```python
from build123d import *

# Parameters (mm, degrees)
SKETCH1_R               = 6.35
BOSS_EXTRUDE1_DEPTH     = 17.5
CUT_EXTRUDE1_DEPTH      = 13
CHAMFER1_SIZE           = 2
SKETCH4_R               = 3.5
BOSS_EXTRUDE2_DEPTH     = 25
SKETCH6_R               = 1.75
CUT_EXTRUDE2_DEPTH      = 30
SKETCH7_R               = 2.5
CUT_EXTRUDE3_DEPTH      = 3.5
CUT_EXTRUDE4_DEPTH      = 101.436547133
CUT_EXTRUDE4_DEPTH_BACK = 101.436547133
SKETCH8_W               = 138.060190548
SKETCH8_H               = 48.357154547
SKETCH9_R               = 6.935
CUT_EXTRUDE5_DEPTH      = 1
MIRROR1_START           = -12.5
MIRROR1_OUTLINE_R       = 1.75
MIRROR1_DEPTH           = 25
MIRROR1_START_2         = -17.5
MIRROR1_2_OUTLINE_R     = 2.5
MIRROR1_2_DEPTH         = 3.5
MIRROR1_START_3         = -14
MIRROR1_3_OUTLINE_R     = 1.75
MIRROR1_3_DEPTH         = 1.5
MIRROR1_4_OUTLINE_R     = 6.935
MIRROR1_4_OUTLINE_R_2   = 6.35
MIRROR1_4_DEPTH         = 1
CUT_EXTRUDE6_DEPTH      = 101.436547133
CUT_EXTRUDE6_DEPTH_BACK = 101.436547133
SKETCH10_W              = 1
SKETCH10_H              = 7.5


# Read off the part's stored shape, not the designer's step: Mirror1
with BuildPart() as part:
    # Sketch1 → Boss-Extrude1 (new, symmetric)
    with BuildSketch(Plane(origin=(0, 0, 0), x_dir=(0, 0, -1), z_dir=(1, 0, 0))):
        with BuildLine():
            Line((-75, -17.5), (75, -17.5))
            ThreePointArc((75, -17.5), (91.201851746, -6.614378278), (87.247448714, 12.5))
            Line((87.247448714, 12.5), (-87.247448714, 12.5))
            ThreePointArc((-87.247448714, 12.5), (-91.201851746, -6.614378278), (-75, -17.5))
        make_face()
        with Locations((-75, 0)):
            Circle(SKETCH1_R, mode=Mode.SUBTRACT)
        with Locations((75, 0)):
            Circle(SKETCH1_R, mode=Mode.SUBTRACT)
    extrude(amount=BOSS_EXTRUDE1_DEPTH, both=True)

    # Sketch3 → Cut-Extrude1 (cut, symmetric)
    with BuildSketch(Plane(origin=(0, 0, 0), x_dir=(0, 0, -1), z_dir=(1, 0, 0))):
        with BuildLine():
            Line((-92.5, 12.5), (75, 12.5))
            ThreePointArc((75, 12.5), (87.5, 0), (75, -12.5))
            Line((75, -12.5), (-55, -12.5))
            Line((-55, -12.5), (-55, -17.5))
            Line((-55, -17.5), (-92.5, -17.5))
            Line((-92.5, -17.5), (-92.5, 12.5))
        make_face()
    extrude(amount=CUT_EXTRUDE1_DEPTH, both=True, mode=Mode.SUBTRACT)

    # Chamfer1
    chamfer1_edges = [part.edges().sort_by_distance(p)[0] for p in [
        (17.5, -6.614378278, -91.201851746),
        (0, -12.5, 55),
        (17.5, -6.614378278, 91.201851746),
        (-17.5, -6.614378278, -91.201851746),
        (-17.5, -17.5, 0),
        (-17.5, -6.614378278, 91.201851746),
        (17.5, -17.5, 0),
    ]]
    chamfer(chamfer1_edges, length=CHAMFER1_SIZE)

    # Sketch4 → Boss-Extrude2 (add)
    with BuildSketch(Plane(origin=(0, -12.5, 0), x_dir=(1, 0, 0), z_dir=(0, 1, 0))):
        with Locations((-10, 62.5)):
            Circle(SKETCH4_R)
        with Locations((-10, 26.333333333)):
            Circle(SKETCH4_R)
        with Locations((-10, -9.833333333)):
            Circle(SKETCH4_R)
        with Locations((-10, -46)):
            Circle(SKETCH4_R)
    extrude(amount=BOSS_EXTRUDE2_DEPTH)

    # Sketch6 → Cut-Extrude2 (cut)
    with BuildSketch(Plane(origin=(0, 12.5, 0), x_dir=(1, 0, 0), z_dir=(0, 1, 0))):
        with Locations(Location((-10, 62.5, 0), (0, 0, 270))):
            Circle(SKETCH6_R)
        with Locations(Location((-10, 26.333333333, 0), (0, 0, 270))):
            Circle(SKETCH6_R)
        with Locations(Location((-10, -9.833333333, 0), (0, 0, 270))):
            Circle(SKETCH6_R)
        with Locations(Location((-10, -46, 0), (0, 0, 270))):
            Circle(SKETCH6_R)
    extrude(amount=-CUT_EXTRUDE2_DEPTH, mode=Mode.SUBTRACT)

    # Sketch7 → Cut-Extrude3 (cut)
    with BuildSketch(Plane.XZ.offset(17.5)):
        with Locations(Location((-10, 46, 0), (0, 0, 270))):
            Circle(SKETCH7_R)
        with Locations(Location((-10, 9.833333333, 0), (0, 0, 270))):
            Circle(SKETCH7_R)
        with Locations(Location((-10, -26.333333333, 0), (0, 0, 270))):
            Circle(SKETCH7_R)
        with Locations(Location((-10, -62.5, 0), (0, 0, 270))):
            Circle(SKETCH7_R)
    extrude(amount=-CUT_EXTRUDE3_DEPTH, mode=Mode.SUBTRACT)

    # Sketch8 → Cut-Extrude4 (cut, two sides: drawn at the far end of the back side and taken through both)
    with BuildSketch(Plane(origin=(17.5, 0, 0), x_dir=(0, 0, -1), z_dir=(1, 0, 0)).offset(-CUT_EXTRUDE4_DEPTH_BACK)):
        with Locations((34.687663788, -4.667734514)):
            Rectangle(SKETCH8_W, SKETCH8_H)
    extrude(amount=CUT_EXTRUDE4_DEPTH + CUT_EXTRUDE4_DEPTH_BACK, mode=Mode.SUBTRACT)

    # Sketch9 → Cut-Extrude5 (cut)
    with BuildSketch(Plane.ZY.offset(-13)):
        with Locations((75, 0)):
            Circle(SKETCH9_R)
    extrude(amount=-CUT_EXTRUDE5_DEPTH, mode=Mode.SUBTRACT)

    # Mirror1 outline → Mirror1 (add)
    with BuildSketch(Plane(origin=(0, 0, 0), x_dir=(1, 0, 0), z_dir=(0, 1, 0)).offset(MIRROR1_START)):
        with BuildLine():
            ThreePointArc((13, -44.197224362), (6.5, -46), (13, -47.802775638))
            Line((13, -47.802775638), (13, -44.197224362))
        make_face()
        with Locations((10, -46)):
            Circle(MIRROR1_OUTLINE_R, mode=Mode.SUBTRACT)
    extrude(amount=MIRROR1_DEPTH)

    # Mirror1 2 outline → Mirror1 2 (cut)
    with BuildSketch(Plane(origin=(0, 0, 0), x_dir=(1, 0, 0), z_dir=(0, 1, 0)).offset(MIRROR1_START_2)):
        with Locations((10, -46)):
            Circle(MIRROR1_2_OUTLINE_R)
    extrude(amount=MIRROR1_2_DEPTH, mode=Mode.SUBTRACT)

    # Mirror1 3 outline → Mirror1 3 (cut)
    with BuildSketch(Plane(origin=(0, 0, 0), x_dir=(1, 0, 0), z_dir=(0, 1, 0)).offset(MIRROR1_START_3)):
        with Locations((10, -46)):
            Circle(MIRROR1_3_OUTLINE_R)
    extrude(amount=MIRROR1_3_DEPTH, mode=Mode.SUBTRACT)

    # Mirror1 4 outline → Mirror1 4 (cut)
    with BuildSketch(Plane.YZ.offset(MIRROR1_START_3)):
        with Locations((0, 75)):
            Circle(MIRROR1_4_OUTLINE_R)
        with Locations((0, 75)):
            Circle(MIRROR1_4_OUTLINE_R_2, mode=Mode.SUBTRACT)
    extrude(amount=MIRROR1_4_DEPTH, mode=Mode.SUBTRACT)

    # Sketch10 → Cut-Extrude6 (cut, two sides: drawn at the far end of the back side and taken through both)
    with BuildSketch(Plane.ZY.offset(17.5).offset(-CUT_EXTRUDE6_DEPTH_BACK)):
        with Locations((75, 3.75)):
            Rectangle(SKETCH10_W, SKETCH10_H)
    extrude(amount=CUT_EXTRUDE6_DEPTH + CUT_EXTRUDE6_DEPTH_BACK, mode=Mode.SUBTRACT)


solid = part.part
```
Input: part model. Units: mm. Frame: model coordinates. A direction names the side the tool comes from. Coordinates: 2 decimals unless noted, no trailing zeros. Write each loop counter-clockwise with the first axis right and the second up, starting at its lowest first coordinate (ties: lowest second). Pieces come first, ordered by that corner, then holes. Notation, with made-up numbers: (74.5, -36) - (106.5, -36) arc R23 cw to (106.5, -15) - close; hole circle Ø8 at (48, -20). An arc over 180 degrees is marked (long way). Put each result on its own line as item: value. Start each with the question number.
1) Cut plane B-B (z = 46). Return the cut outline in (x, y).
2) Reachability of faces 5 (the face through (-13, 0, 39)), 6 (the face through (-14, 3, 69)), 7 (the face through (9.46, -15.77, 48.44)), 8 (the face through (0.2, -13.5, 54)), 9 (the face through (14, 12.5, 60)) from +Z, -Z, +X, -X, +Y, -Y: full face, straight path, thin tool, end or side. Return the list, or none.
3) Mould query, pull axis Z, two halves, no side actions, for faces 1 (the face through (0, -13, 34.342)), 2 (the face through (13.49, -6.93, 74.7)), 3 (the face through (17.5, -1, 63)), 4 (the face through (9.62, -0.94, 47.71)). Classes: pulls with the +Z half, pulls with the -Z half, needs draft (parallel to the pull), parting line crosses it, or undercut.
4) Contact query for flat-ended pins moving along their axis: pin 1 (10 mm diameter, centred on y = 0, z = 75, fed in from -X); pin 2 (1 mm diameter, centred on x = 6.5, y = 5, fed in from +Z); pin 3 (3.5 mm diameter, centred on x = 3, y = -16, fed in from +Z); pin 4 (1.5 mm diameter, centred on x = 11, y = 7, fed in from +Z). Output: stop coordinate, or through.
5) Cut plane C-C (x = 10). Return the cut outline in (y, z).
6) Cut plane D-D (y = 3). State how many separate pieces and enclosed holes the cut face has, plus the area to 3 significant figures.
7) Ray query, L1, parallel to X at y = -4, z = 61; L2, parallel to Z at x = 10, y = 5; L3, parallel to Y at x = -15, z = 75. Return the intervals inside material, ascending.
8) Cut plane A-A (z = 63.5). Return the cut outline in (x, y), plus the area to 3 significant figures.
Resolved:
1. outline: (-17.5, -15.5) - (-15.5, -17.5) - (-12.5, -17.5) - (-12.5, -14) - (-11.75, -14) - (-11.75, 12.5) - (-17.5, 12.5) - close; (-8.25, -14) - (-7.5, -14) - (-7.5, -17.5) - (7.5, -17.5) - (7.5, -14) - (8.25, -14) - (8.25, 12.5) - (6.5, 12.5) - (6.5, -12.5) - (-6.5, -12.5) - (-6.5, 12.5) - (-8.25, 12.5) - close; (11.75, -14) - (12.5, -14) - (12.5, -17.5) - (15.5, -17.5) - (17.5, -15.5) - (17.5, 12.5) - (11.75, 12.5) - close
2. face 5: -Z, +Y
2. face 6: none
2. face 7: -Y
2. face 8: +Z, +Y
2. face 9: +Z, -Z, +X, -X, +Y
3. face 1: pulls with the -Z half
3. face 2: undercut
3. face 3: needs draft
3. face 4: undercut
4. pin 1: passes through
4. pin 2: stops at z = 47.8
4. pin 3: stops at z = 55
4. pin 4: stops at z = 49.49
5. outline: (-17.5, 34.34) - (-12.5, 34.34) - (-12.5, 42.5) - (12.5, 42.5) - (12.5, 44.25) - (-14, 44.25) - (-14, 43.5) - (-17.5, 43.5) - close; (-17.5, 48.5) - (-14, 48.5) - (-14, 47.75) - (12.5, 47.75) - (12.5, 49.5) - (-12.5, 49.5) - (-12.5, 53) - (-14.5, 55) - (-17.5, 55) - close
6. separate pieces: 4
6. enclosed holes: 2
6. area: 469 mm2
7. L1: x = -17.5 to -13, 13 to 17.5
7. L2: z = 42.5 to 44.25, 47.75 to 49.5
7. L3: y = -17.5 to -6.35, 7.5 to 12.5
8. outline: (-17.5, -15.5) - (-15.5, -17.5) - (-13, -17.5) - (-13, 12.5) - (-17.5, 12.5) - close; (13, -17.5) - (15.5, -17.5) - (17.5, -15.5) - (17.5, 12.5) - (13, 12.5) - close
8. area: 266 mm2
